Geometry check sheet. Reference: the model listing, model coordinates, mm. A direction names the side the tool comes from. Round coordinates to 2 decimals unless told otherwise and drop trailing zeros. Write each loop counter-clockwise with the first axis right and the second up, starting at its lowest first coordinate (ties: lowest second). Pieces come first, ordered by that corner, then holes.
from build123d import *

# Parameters (mm, degrees)
CROQUIS1_W              = 203.2
CROQUIS1_H              = 38.1
SALIENTE_EXTRUIR2_DEPTH = 38.1
CROQUIS2_R              = 6.35
SALIENTE_EXTRUIR3_DEPTH = 12.7
CROQUIS3_R              = 6.35
SALIENTE_EXTRUIR4_DEPTH = 12.7


with BuildPart() as part:
    # Croquis1 → Saliente-Extruir2 (new body)
    with BuildSketch(Plane(origin=(0, 0, 0), x_dir=(1, 0, 0), z_dir=(0, 1, 0))):
        Rectangle(CROQUIS1_W, CROQUIS1_H)
    extrude(amount=SALIENTE_EXTRUIR2_DEPTH)

    # Croquis2 → Saliente-Extruir3 (add)
    with BuildSketch(Plane(origin=(101.6, 0, 0), x_dir=(0, 0, -1), z_dir=(1, 0, 0))):
        with Locations((0, 19.05)):
            Circle(CROQUIS2_R)
    extrude(amount=SALIENTE_EXTRUIR3_DEPTH)

    # Croquis3 → Saliente-Extruir4 (add)
    with BuildSketch(Plane.ZY.offset(101.6)):
        with Locations((0, 19.05)):
            Circle(CROQUIS3_R)
    extrude(amount=SALIENTE_EXTRUIR4_DEPTH)


solid = part.part
1. Depth check by flat-ended pin: pin 1 Ø4 at (y, z) = (27.5, 10.5) entering from +X; pin 2 Ø10 at (y, z) = (8, 10.5) entering from -X. Enter the tip coordinate at first touch or a pass-through.
2. Access from +Z, -Z, +X, -X, +Y, -Y to the whole of each face (thin tool, end or side, straight path). Record for faces 1 (the face through (-1, 19, -19.05)), 2 (the face through (-101.6, 19, 9)), 3 (the face through (101.6, 19, 9)).
3. Section check A-A (y = 19.05). Record the cut outline in (x, z).
4. Section check B-B (z = 0). Record the cut outline in (x, y), plus the area to 3 significant figures.
5. Section check D-D (y = 10.5). Record the cut outline in (x, z).
6. Section check C-C (z = -17). Record the cut outline in (x, y), plus the area to 3 significant figures.
7. Scan lines: line 1 along X through (y, z) = (9, 9); line 2 along Z through (x, y) = (-104, 19). Record each from-to range of solid material in increasing order.
Results below:
1. pin 1: stops at x = 101.6
1. pin 2: stops at x = -101.6
2. face 1: -Z, +X, -X, +Y, -Y
2. face 2: -X
2. face 3: +X
3. outline: (-114.3, -6.35) - (-101.6, -6.35) - (-101.6, -19.05) - (101.6, -19.05) - (101.6, -6.35) - (114.3, -6.35) - (114.3, 6.35) - (101.6, 6.35) - (101.6, 19.05) - (-101.6, 19.05) - (-101.6, 6.35) - (-114.3, 6.35) - close
4. outline: (-114.3, 12.7) - (-101.6, 12.7) - (-101.6, 0) - (101.6, 0) - (101.6, 12.7) - (114.3, 12.7) - (114.3, 25.4) - (101.6, 25.4) - (101.6, 38.1) - (-101.6, 38.1) - (-101.6, 25.4) - (-114.3, 25.4) - close
4. area: 8,060 mm2
5. outline: (-101.6, -19.05) - (101.6, -19.05) - (101.6, 19.05) - (-101.6, 19.05) - close
6. outline: (-101.6, 0) - (101.6, 0) - (101.6, 38.1) - (-101.6, 38.1) - close
6. area: 7,740 mm2
7. line 1: x = -101.6 to 101.6
7. line 2: z = -6.35 to 6.35
